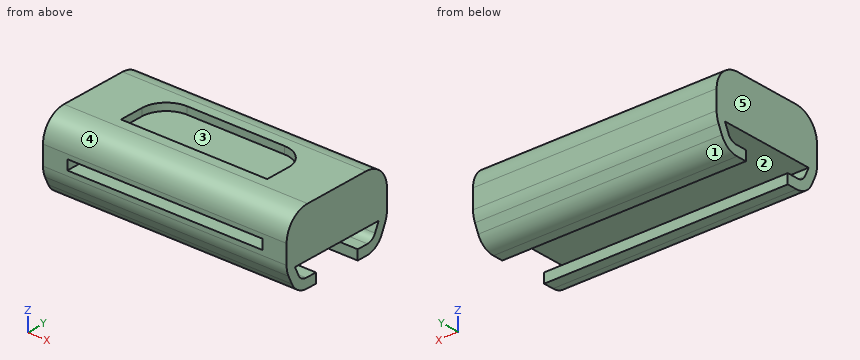
from build123d import *

# Parameters (mm, degrees)
F0_W      = 50
F0_H      = 24
F1_DEPTH  = 10
F3_DEPTH  = 50
F4_R      = 5
F5_R      = 2
F6_R      = 4
F7_W      = 40
F7_H      = 2
F8_DEPTH  = 3
F9_W      = 30
F9_H      = 10
F10_DEPTH = 1.5
F11_R     = 5


with BuildPart() as f1:
    # F0 (on Top) → F1 (new body)
    with BuildSketch(Plane.XY):
        Rectangle(F0_W, F0_H)
    extrude(amount=F1_DEPTH)

    # F2 (on face) → F3 (join, through all)
    with BuildSketch(Plane(origin=(-25, 0, 0), x_dir=(0, -1, 0), z_dir=(-1, 0, 0))):
        Polygon((-10, 0), (-12, 0), (-9.673886, -5), (-5, -5), (-5, -3), (-8.604331, -3), align=None)
        Polygon((12, 0), (10, 0), (8.604331, -3), (5, -3), (5, -5), (9.673886, -5), align=None)
    extrude(amount=-F3_DEPTH)

    # F4
    f4_edges = [f1.edges().sort_by_distance(p)[0] for p in [
        (0, 12, 10),
        (0, -12, 10),
        (0, 12, 0),
        (0, -12, 0),
    ]]
    fillet(f4_edges, radius=F4_R)

    # F5
    f5_edges = [f1.edges().sort_by_distance(p)[0] for p in [
        (0, 8.604331, -3),
        (0, -8.604331, -3),
    ]]
    fillet(f5_edges, radius=F5_R)

    # F6
    f6_edges = [f1.edges().sort_by_distance(p)[0] for p in [
        (0, 9.673886, -5),
        (0, -9.673886, -5),
    ]]
    fillet(f6_edges, radius=F6_R)

    # F7 (on face) → F8 (cut)
    with BuildSketch(Plane.XZ.offset(12)):
        with Locations((0, 3.088876)):
            Rectangle(F7_W, F7_H)
    extrude(amount=-F8_DEPTH, mode=Mode.SUBTRACT)

    # F9 (on face) → F10 (cut)
    with BuildSketch(Plane.XY.offset(10)):
        Rectangle(F9_W, F9_H)
    extrude(amount=-F10_DEPTH, mode=Mode.SUBTRACT)

    # F11
    f11_edges = [f1.edges().sort_by_distance(p)[0] for p in [
        (-15, 5, 9.25),
        (15, 5, 9.25),
    ]]
    fillet(f11_edges, radius=F11_R)


solid = f1.part
Input: part model. Units: mm. Frame: model coordinates. Face numbers are marked on the shaded views. A direction names the side the tool comes from. Coordinates: 2 decimals unless noted, no trailing zeros. Loops run counter-clockwise (first coordinate to the right, second up) from the corner with the lowest first, then second, coordinate; pieces in that order, holes last.
(1) Section A-A on x = 18. Return the cut outline in (y, z), then the cut area to 3 significant figures.
(2) Section C-C on z = 3.5. Return the cut outline in (x, y), then the cut area to 3 significant figures.
(3) First-contact query: pin 1 Ø2.5 at (x, y) = (0, -10.5) entering from -Z; pin 2 Ø1.5 at (x, y) = (6.5, -10) entering from +Z; pin 3 Ø1 at (x, z) = (12, -4.5) entering from +Y; pin 4 Ø6 at (y, z) = (9, -1) entering from -X. Flat tips, straight axial feed; report the tip coordinate or a pass-through.
(4) Section D-D on z = -3.5. Return the cut outline in (x, y), then the cut area to 3 significant figures.
(5) Section B-B on y = 8. Return the cut outline in (x, z), then the cut area to 3 significant figures.
(6) Pull-direction query (X, two-part tool) for the marked faces 3, 4 and 5; classes: released by +X, released by -X, zero draft, split by the parting line, or undercut.
(7) Material intervals for probe 1 along Z at (x, y) = (-9, -7); probe 2 along X at (y, z) = (-2, 9.25); probe 3 along Z at (x, y) = (-4, 1), sorted ascending.
(8) Set-up query: the marked faces 1 and 2. Return all of +Z, -Z, +X, -X, +Y, -Y with unobstructed straight access to the full face (end or side cutting, diameter ignored); none if empty.
Data:
1. outline: (-12, 1.11) arc R5 ccw to (-11.53, -1) - (-10.75, -2.69) arc R4 ccw to (-7.12, -5) - (-5, -5) - (-5, -3) - (-7.33, -3) arc R2 cw to (-9.14, -1.84) - (-10, 0) - (10, 0) - (9.14, -1.84) arc R2 cw to (7.33, -3) - (5, -3) - (5, -5) - (7.12, -5) arc R4 ccw to (10.75, -2.69) - (11.53, -1) arc R5 ccw to (12, 1.11) - (12, 5) arc R5 ccw to (7, 10) - (-7, 10) arc R5 ccw to (-12, 5) - (-12, 4.09) - (-9, 4.09) - (-9, 2.09) - (-12, 2.09) - close
1. area: 254 mm2
2. outline: (-25, -12) - (-20, -12) - (-20, -9) - (20, -9) - (20, -12) - (25, -12) - (25, 12) - (-25, 12) - close
2. area: 1,080 mm2
3. pin 1: stops at z = -4.39
3. pin 2: stops at z = 9.47
3. pin 3: stops at y = 9.77
3. pin 4: stops at x = -25
4. outline: (-25, -10.25) - (25, -10.25) - (25, -5) - (-25, -5) - close; (-25, 5) - (25, 5) - (25, 10.25) - (-25, 10.25) - close
4. area: 525 mm2
5. outline: (-25, -4.9) - (25, -4.9) - (25, -2.88) - (-25, -2.88) - close; (-25, 0) - (25, 0) - (25, 9.9) - (-25, 9.9) - close
5. area: 596 mm2
6. face 3: undercut
6. face 4: zero draft
6. face 5: released by -X
7. probe 1: z = -5 to -3, 0 to 10
7. probe 2: x = -25 to -15, 15 to 25
7. probe 3: z = 0 to 8.5
8. face 1: -Z, +X, -X, +Y
8. face 2: +X, -X
